Check sheet for the modelled part. Datum: model origin and axes. Units: mm. Round coordinates to 2 decimals unless told otherwise and drop trailing zeros. Order: outer loops, then holes, each group sorted by start corner. A loop starts at its lowest first (then second) coordinate and runs counter-clockwise, first axis right, second up. Notation, with made-up numbers: (-21, -7) -> (17, -7) arc R23 cw to (17, 29) -> close; hole circle Ø8 at (57.5, 28). An arc over 180 degrees is marked (long way). Use CSV: the item, a comma, the result in double quotes.
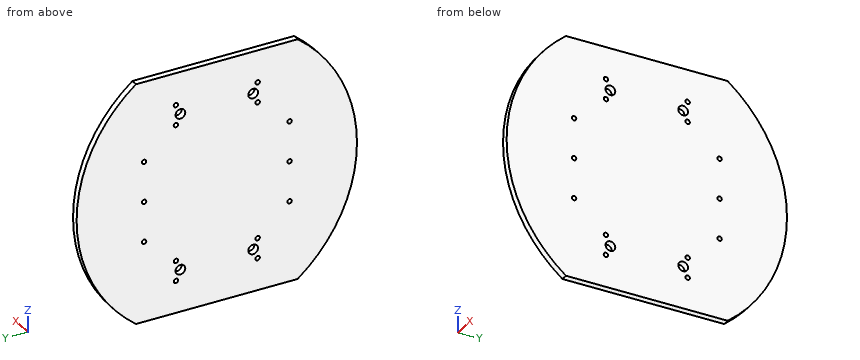
```python
from build123d import *

# Parameters (mm, degrees)
EXTRUDE_1_DEPTH     = 8
SKETCH_2_R          = 6
SKETCH_2_R_2        = 2.75
CUT_EXTRUDE_1_DEPTH = 8
SKETCH_3_R          = 2.75
CUT_EXTRUDE_2_DEPTH = 10


with BuildPart() as part:
    # 草图1 → 凸台-拉伸1 (new body)
    with BuildSketch(Plane(origin=(0, 0, 0), x_dir=(0, 0, -1), z_dir=(1, 0, 0))):
        with BuildLine():
            Line((-150, 100), (-150, -100))
            ThreePointArc((-150, -100), (0, -173.380962103), (150, -100))
            Line((150, -100), (150, 100))
            ThreePointArc((150, 100), (0, 173.380962103), (-150, 100))
        make_face()
    extrude(amount=EXTRUDE_1_DEPTH)

    # 草图2 → 切除-拉伸1 (cut)
    with BuildSketch(Plane(origin=(8, 0, 0), x_dir=(0, 0, -1), z_dir=(1, 0, 0))):
        with Locations((97.5, 45)):
            Circle(SKETCH_2_R)
        with Locations((97.5, -45)):
            Circle(SKETCH_2_R)
        with Locations((85, 50.5)):
            Circle(SKETCH_2_R_2)
        with Locations((110, 50.5)):
            Circle(SKETCH_2_R_2)
        with Locations((85, -50.5)):
            Circle(SKETCH_2_R_2)
        with Locations((110, -50.5)):
            Circle(SKETCH_2_R_2)
        with Locations(Location((-110, -50.5, 0), (0, 0, 180))):
            Circle(SKETCH_2_R_2)
        with Locations(Location((-85, -50.5, 0), (0, 0, 180))):
            Circle(SKETCH_2_R_2)
        with Locations(Location((-110, 50.5, 0), (0, 0, 180))):
            Circle(SKETCH_2_R_2)
        with Locations(Location((-85, 50.5, 0), (0, 0, 180))):
            Circle(SKETCH_2_R_2)
        with Locations(Location((-97.5, -45, 0), (0, 0, 180))):
            Circle(SKETCH_2_R)
        with Locations(Location((-97.5, 45, 0), (0, 0, 180))):
            Circle(SKETCH_2_R)
    extrude(amount=-CUT_EXTRUDE_1_DEPTH, mode=Mode.SUBTRACT)

    # 草图3 → 切除-拉伸2 (cut)
    with BuildSketch(Plane(origin=(8, 0, 0), x_dir=(0, 0, -1), z_dir=(1, 0, 0))):
        with Locations((-50, 90)):
            Circle(SKETCH_3_R)
        with Locations((0, 90)):
            Circle(SKETCH_3_R)
        with Locations((50, 90)):
            Circle(SKETCH_3_R)
        with Locations((50, -90)):
            Circle(SKETCH_3_R)
        with Locations((0, -90)):
            Circle(SKETCH_3_R)
        with Locations((-50, -90)):
            Circle(SKETCH_3_R)
    extrude(amount=-CUT_EXTRUDE_2_DEPTH, mode=Mode.SUBTRACT)


solid = part.part
```
Q1. Go/stop test with flat-tipped pins: pin 1 (6.5 mm diameter, centred on y = -50.5, z = -85, fed in from +X); pin 2 (5 mm diameter, centred on y = 50.5, z = -85, fed in from +X); pin 3 (4 mm diameter, centred on x = 6, y = -120.5, fed in from +Z); pin 4 (1.5 mm diameter, centred on x = 2, z = -42, fed in from +Y). Record where each tip stops, or that it passes through.
Result sheet:
pin 1,"stops at x = 8"
pin 2,"passes through"
pin 3,"stops at z = 133.58"
pin 4,"stops at y = 168.85"
Q2. Sectioned sample at C-C, the plane y = -117. Enter the section's corners in (x, z).
Result sheet:
outline,"(0, -135.08) -> (8, -135.08) -> (8, 135.08) -> (0, 135.08) -> close"
Q3. Scan lines: L1, parallel to Y at x = 2, z = 0; L2, parallel to Y at x = 3, z = -110; L3, parallel to Z at x = 0.5, y = -89. Record each from-to range of solid material in increasing order.
Result sheet:
L1,"y = -173.38 to -92.75, -87.25 to 87.25, 92.75 to 173.38"
L2,"y = -138.3 to -53.25, -47.75 to 47.75, 53.25 to 138.3"
L3,"z = -150 to -52.56, -47.44 to -2.56, 2.56 to 47.44, 52.56 to 150"
Q4. Sectioned sample at A-A, the plane x = 1.25. State how many separate pieces and enclosed holes the cut face has, then the cut area to 3 significant figures.
Result sheet:
separate pieces,"1"
enclosed holes,"18"
area,"89,900 mm^2"
Q5. Sectioned sample at B-B, the plane z = -42. Enter the section's corners in (x, y).
Result sheet:
outline,"(0, -168.68) -> (8, -168.68) -> (8, 168.68) -> (0, 168.68) -> close"
